Geometry check sheet. Reference: the model listing, model coordinates, mm. A direction names the side the tool comes from. Coordinates: 2 decimals unless noted, no trailing zeros. Write each loop counter-clockwise with the first axis right and the second up, starting at its lowest first coordinate (ties: lowest second). Pieces come first, ordered by that corner, then holes. Notation, with made-up numbers: M 80,68 L 93,68 A20 cw 93,86 Z; hole C 72.5,8 d2. An arc over 180 degrees is marked long. Put each result on its own line as item: value. Start each with the question number.
1) Mould release check, pull along Y, two halves, no side actions. Record for faces 3 (the flat face through (-8, 8, -3)), 4 (the flat face through (0, 6, -1)), 5 (the flat face through (-4, 4, 0)): released by +Y, released by -Y, zero draft, split by the parting line, or undercut.
2) Cross-section at D-D on x = -7. Record the cut outline in (y, z), plus the area to 3 significant figures.
3) Cross-section at B-B on z = -7.75. Record the cut outline in (x, y), plus the area to 3 significant figures.
4) Gauge pin test, flat ends, axial feed: pin 1 (1.5 mm diameter, centred on y = 4, z = -8.5, fed in from +X); pin 2 (1.5 mm diameter, centred on x = -6, y = 3.5, fed in from -Z). Record the tip position at first contact, or that the pin passes through.
5) Cross-section at C-C on y = 3.25. Record the cut outline in (x, z), plus the area to 3 significant figures.
6) Set-up check for faces 1 (the flat face through (-6, 5.5, -6)), 2 (the cylindrical face through (-12.323, 3.929, 1.014)): record each of +Z, -Z, +X, -X, +Y, -Y from which the full face is reachable in a straight line by a thin tool's end or side.
7) Scan lines: line 1 along Y through (x, z) = (-9.75, -3.5); line 2 along Z through (x, y) = (-11, 7); line 3 along X through (y, z) = (1.75, 0). Record each from-to range of solid material in increasing order.
8) Cross-section at A-A on y = 1.5. Record the cut outline in (x, z), plus the area to 3 significant figures.
Autodesk Inventor part; units mm, degrees
ref_plane "Work Plane1" through (0, 5.5, 0) normal (0, 1, 0) x (1, 0, 0)
ref_plane "YZ Plane" through (0, 0, 0) normal (1, 0, 0) x (0, 1, 0)
ref_plane "XZ Plane" through (0, 0, 0) normal (0, 1, 0) x (-1, 0, 0)
sketch "Sketch1" plane through (0, 0, 0) normal (0, 1, 0) x (-1, 0, 0)
  line L0 (0, 0) -> (8, 0)
  line L1 (0, 0) -> (0, 5)
  line L2 (0, 5) -> (16, 5)
  arc A0 (11, -3) -> (8, 0) centre (8, -3) ccw
  line L3 (11, -3) -> (11, -11)
  line L4 (11, -11) -> (16, -11)
  line L5 (16, -11) -> (16, 5)
  line L6 (0, 0) -> (11, -11)
  dimension "d0" = 5
  dimension "d1" = 5
  dimension "d2" = 8
  dimension "d3" = 3
  dimension "d4" = 8
extrude "Extrusion1" add sketch "Sketch1" along normal blind 8 contours L1 L2 L5 L4 L3 A0 L0
sketch "Sketch2" plane through (0, 0, 0) normal (0, -1, 0) x (1, 0, 0)
  line L0 (0, 0) -> (-8, 0)
  arc A0 (-8, 0) -> (-11, -3) centre (-8, -3) ccw
  line L1 (-11, -3) -> (-11, -11)
  line L2 (0, 0) -> (-11, -11)
  line L3 (-11, -11) -> (-11, -3)
  line L4 (-8, 0) -> (0, 0)
  arc A1 (-8, 0) -> (-11, -3) centre (-8, -3) ccw
  line L5 (0, 0) -> (0, -8)
  arc A2 (-3, -11) -> (0, -8) centre (-3, -8) ccw
  line L6 (-3, -11) -> (-11, -11)
extrude "Extrusion2" add sketch "Sketch2" against normal blind 2.5
ref_plane "Work Plane1" through (0, 5.5, 0) normal (0, 1, 0) x (1, 0, 0)
sketch "Sketch3" plane through (0, 5.5, 0) normal (0, 1, 0) x (1, 0, 0)
  line L0 (0, 0) -> (0, 8)
  arc A0 (0, 8) -> (-3, 11) centre (-3, 8) ccw
  line L1 (-3, 11) -> (-11, 11)
  line L2 (-11, 3) -> (-11, 11)
  arc A1 (-11, 3) -> (-8, 0) centre (-8, 3) ccw
  line L3 (0, 0) -> (-8, 0)
extrude "Extrusion3" add sketch "Sketch3" along normal blind 2.5
sketch "Sketch4" plane through (0, 8, 0) normal (0, 1, 0) x (1, 0, 0)
  arc A0 (0, 8) -> (-3, 11) centre (-3, 8) ccw
  line L0 (0, -5) -> (0, 8)
  line L1 (-3, 11) -> (-16, 11)
  line L2 (-16, 11) -> (-16, -5)
  line L3 (-16, -5) -> (0, -5)
  point P0 (0, 0)
sketch "Sketch5" plane through (0, 8, 0) normal (0, 1, 0) x (1, 0, 0)
  circle A0 centre (-11, 0) radius 1.6667
  line L0 (-16, -5) -> (0, -5)
  line L1 (-16, 11) -> (-16, -5)
  point P0 (0, 0)
  point P1 (-8, -5)
  point P2 (-16, 3)
  dimension "d21" = 3.3333
  dimension "d22" = 3.3333
  dimension "d23" = 3.3333
extrude "Extrusion4" cut sketch "Sketch5" against normal through all
fillet "Fillet2" radius 0.25 1 edges at (-12.6667, 8, 0)
fillet "Fillet3" radius 4 1 edges at (-16, 4, 5)
equation "\"d1\" = d0"
equation "\"d23\" = d22"
properties part number "Plate Adapter 5.0"
Answer key:
1. face 3: released by +Y
1. face 4: zero draft
1. face 5: undercut
2. outline: M 0,-11 L 2.5,-11 L 2.5,0 L 5.5,0 L 5.5,-11 L 8,-11 L 8,5 L 0,5 Z
2. area: 95.0 mm²
3. outline: M -16,0 L 0,0 L 0,2.5 L -11,2.5 L -11,5.5 L 0,5.5 L 0,8 L -16,8 Z
3. area: 95.0 mm²
4. pin 1: stops at x = -11
4. pin 2: stops at z = 0
5. outline: M -16,-11 L -11,-11 L -11,-3 A3 cw -10.67,-1.63 A1.67 cw long -9.37,-0.33 A3 cw -8,0 L 0,0 L 0,5 L -12,5 A4 ccw -16,1 Z
5. area: 125 mm²
6. face 1: -Z, +X
6. face 2: +Y, -Y
7. line 1: y = 0 to 2.5, 5.5 to 8
7. line 2: z = -11 to -1.67, 1.67 to 5
7. line 3: x = -16 to -12.67, -9.33 to 0
8. outline: M -16,-11 L -3,-11 A3 ccw 0,-8 L 0,5 L -12,5 A4 ccw -16,1 Z; hole C -11,0 d3.33
8. area: 242 mm²
